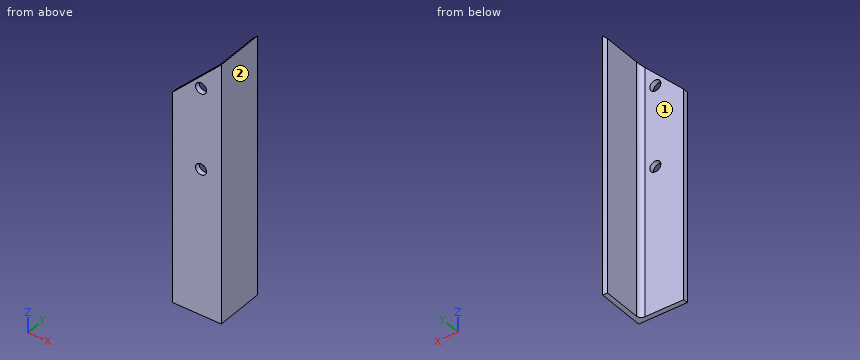
```python
from build123d import *

# Parameters (mm, degrees)
F1_DEPTH = 160
F2_R     = 3
F4_DEPTH = 30.001
F6_D     = 6.8


with BuildPart() as f1:
    # F0 (on Top) → F1 (new body)
    with BuildSketch(Plane.XY):
        Polygon((0, 3), (0, 0), (30, 0), (30, 30), (27, 30), (27, 3), align=None)
    extrude(amount=F1_DEPTH)

    # F2
    f2_edges = [f1.edges().sort_by_distance(p)[0] for p in [
        (27, 3, 80),
    ]]
    fillet(f2_edges, radius=F2_R)

    # F3 (on face) → F4 (cut, through all)
    with BuildSketch(Plane.XZ):
        Polygon((-10, 120), (40, 170), (-10, 170), align=None)
    extrude(amount=-F4_DEPTH, mode=Mode.SUBTRACT)

    # F6 (through all)
    with Locations(Plane.XZ):
        with Locations((17.5, 140), (17.5, 90)):
            Hole(F6_D / 2)


solid = f1.part
```
For this review, take the finished solid that the model builds, in its own axes (mm). Face numbers are marked on the shaded views. A direction names the side the tool comes from. Round coordinates to 2 decimals unless told otherwise and drop trailing zeros. Order: outer loops, then holes, each group sorted by start corner. A loop starts at its lowest first (then second) coordinate and runs counter-clockwise, first axis right, second up. Notation, with made-up numbers: (26, 7) -> (59, 7) arc R28 cw to (59, 40) -> close; hole circle Ø5 at (51.25, 19). An arc over 180 degrees is marked (long way). Use a Markdown table: item, result.
Item 1: Take a section at D-D (y = 27.5). State the section outline as (x, z) points.
Resolved:
| item | result |
|---|---|
| outline | (27, 0) -> (30, 0) -> (30, 160) -> (27, 157) -> close |
Item 2: Machinability: for the marked faces 1 and 2, which of the approach directions +Z, -Z, +X, -X, +Y, -Y give a long, thin tool a straight path to every point of the face, cutting with its end or side? Answer none if there is none.
Resolved:
| item | result |
|---|---|
| face 1 | +Z, -Z, -X, +Y |
| face 2 | +Z, -Z, +X, +Y, -Y |
Item 3: For pin 1 (2 mm diameter, centred on y = 20, z = 98.5, fed in from -X); pin 2 (8 mm diameter, centred on x = 7, y = 4.5, fed in from +Z), all flat-tipped, find the tip position at first contact; note any pin that passes through.
Resolved:
| item | result |
|---|---|
| pin 1 | stops at x = 27 |
| pin 2 | stops at z = 140.71 |
Item 4: Take a section at B-B (z = 140). State the section outline as (x, y) points, plus the area to 3 significant figures.
Resolved:
| item | result |
|---|---|
| outline | (10, 0) -> (14.1, 0) -> (14.1, 3) -> (10, 3) -> close; (20.9, 0) -> (30, 0) -> (30, 30) -> (27, 30) -> (27, 6) arc R3 cw to (24, 3) -> (20.9, 3) -> close |
| area | 123 mm² |
Item 5: Take a section at A-A (x = 17.5). State the section outline as (y, z) points.
Resolved:
| item | result |
|---|---|
| outline | (0, 0) -> (3, 0) -> (3, 86.6) -> (0, 86.6) -> close; (0, 93.4) -> (3, 93.4) -> (3, 136.6) -> (0, 136.6) -> close; (0, 143.4) -> (3, 143.4) -> (3, 147.5) -> (0, 147.5) -> close |
Item 6: For line 1 along Z through (x, y) = (17, 1); line 2 along Z through (x, y) = (20.5, 2); line 3 along X through (y, z) = (17.5, 42.5), list the stretches that pass through material, from the lowest coordinate up. Write a range as [from, to].
Resolved:
| item | result |
|---|---|
| line 1 | z = [0, 86.64], [93.36, 136.64], [143.36, 147] |
| line 2 | z = [0, 88.4], [91.6, 138.4], [141.6, 150.5] |
| line 3 | x = [27, 30] |
Item 7: Take a section at C-C (z = 68.5). State the section outline as (x, y) points, plus the area to 3 significant figures.
Resolved:
| item | result |
|---|---|
| outline | (0, 0) -> (30, 0) -> (30, 30) -> (27, 30) -> (27, 6) arc R3 cw to (24, 3) -> (0, 3) -> close |
| area | 173 mm² |
